Build history of the part. All positions in model axes, mm. Face numbers are marked on the shaded views. A direction names the side the tool comes from. Coordinates: 2 decimals unless noted, no trailing zeros. Loops run counter-clockwise (first coordinate to the right, second up) from the corner with the lowest first, then second, coordinate; pieces in that order, holes last.
(1) Wall check: L1, parallel to Y at x = 35, z = 2.5; L2, parallel to X at y = 50, z = 134; L3, parallel to Y at x = 23, z = 129. Give the ranges that are in metal, low to high.
(2) Slice it at B-B (x = 35). Give the cut face in (y, z).
(3) Two-plate mould, pull along X, no slides. Class the marked faces 4, 5 and 6: pulls with the +X half, pulls with the -X half, needs draft (parallel to the pull), parting line crosses it, or undercut.
(4) Slice it at C-C (z = 112). Give the cut face in (x, y), and give its area (3 significant figures).
(5) Tool access for the marked faces 1, 2 and 3: list every direction of +Z, -Z, +X, -X, +Y, -Y with a clear straight run to the whole face (end or side of a thin tool).
(6) Flat gauge pins, fed straight in: P1, Ø10, axis at x = 7.5, z = 105.5, coming from the +Y side; P2, Ø8, axis at y = 152, z = 72.5, coming from the -X side; P3, Ø24.5, axis at y = 119, z = 119.5, coming from the -X side; P4, Ø6, axis at x = 7, z = 125.5, coming from the +Y side. Where does each tip first touch, or does it go through?
Autodesk Fusion 360 part; units mm, degrees
sketch "Sketch1" plane through (0, 0, 0) normal (0, 1, 0) x (1, 0, 0)
  line L0 (0, 0) -> (70, 0)
  line L1 (70, 0) -> (70, -40)
  line L2 (0, -40) -> (0, 0)
  line L3 (70, -40) -> (12, -40)
  line L4 (70, -90) -> (70, -40)
  line L5 (0, -40) -> (12, -90)
  line L6 (12, -90) -> (12, -140)
  line L7 (12, -140) -> (70, -140)
  line L8 (70, -140) -> (70, -90)
  dimension "d1" = 70
  dimension "d2" = 40
  dimension "d3" = 58
  dimension "d4" = 50
  dimension "d5" = 58
  dimension "d6" = 50
extrude "Extrude1" add sketch "Sketch1" along normal blind 190
sketch "Sketch2" plane through (0, 0, 0) normal (0, 0, -1) x (-1, 0, 0)
  line L0 (-70, 0) -> (0, 0)
  line L1 (0, 0) -> (0, 190)
  line L2 (0, 190) -> (-70, 190)
  line L3 (-70, 190) -> (-70, 0)
sketch "Sketch4" plane through (0, 0, 0) normal (0, 0, -1) x (-1, 0, 0)
  circle A0 centre (-35, 155) radius 25
  line L0 (0, 190) -> (-70, 190)
  line L1 (0, 0) -> (0, 190)
  circle A1 centre (-35, 95) radius 25
  circle A2 centre (-35, 35) radius 25
  dimension "d21" = 50
  dimension "d22" = 35
  dimension "d23" = 35
  dimension "d24" = 50
  dimension "d25" = 35
  dimension "d26" = 60
  dimension "d27" = 50
  dimension "d28" = 35
  dimension "d29" = 60
shell "Shell1" thickness 5 removed faces 1 at (31.3333, 63.3333, 140)
extrude "Extrude2" cut sketch "Sketch4" against normal blind 25
fillet "Fillet1" radius 1 7 edges at (12, 190, 115) (6, 190, 65) (0, 190, 20) (12, 95, 140) (12, 0, 115) (6, 0, 65) (0, 0, 20)
fillet "Fillet2" radius 1 3 edges at (0.2929, 0.2929, 39.9653) (0, 95, 40) (0.2929, 189.7071, 39.9653)
chamfer "Chamfer1" distance 4 angle 45 4 edges at (65, 95, 140) (41, 185, 140) (17, 95, 140) (41, 5, 140)
fillet "Fillet3" radius 0.5 6 edges at (70, 95, 0) (35.5, 190, 0) (0.2929, 189.7071, 0) (0, 95, 0) (0.2929, 0.2929, 0) (35.5, 0, 0)
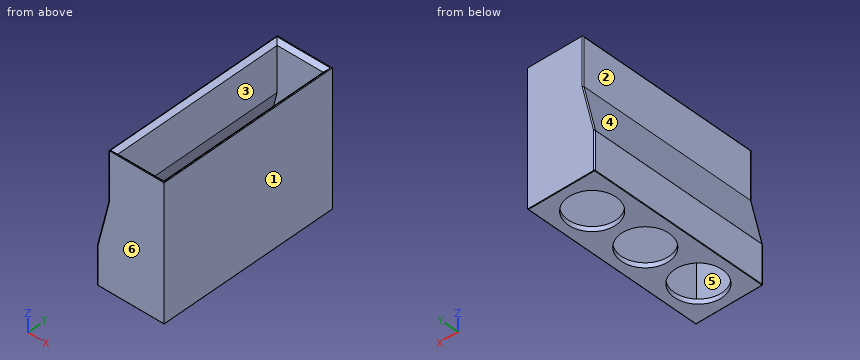
Response values:
1. L1: y = 0 to 10, 60 to 70, 120 to 130, 180 to 190
1. L2: x = 12 to 17, 65 to 70
1. L3: y = 0 to 5, 185 to 190
2. outline: (0, 0.5) arc R0.5 ccw to (0.5, 0) - (10, 0) - (10, 5) - (5, 5) - (5, 136) - (1, 140) - (0, 140) - close; (60, 0) - (70, 0) - (70, 5) - (60, 5) - close; (120, 0) - (130, 0) - (130, 5) - (120, 5) - close; (180, 0) - (189.5, 0) arc R0.5 ccw to (190, 0.5) - (190, 140) - (189, 140) - (185, 136) - (185, 5) - (180, 5) - close
3. face 4: pulls with the -X half
3. face 5: undercut
3. face 6: needs draft
4. outline: (12, 1) arc R1 ccw to (13, 0) - (70, 0) - (70, 190) - (13, 190) arc R1 ccw to (12, 189) - close; hole (17, 5) - (65, 5) - (65, 185) - (17, 185) - close
4. area: 2,380 mm2
5. face 1: +Z, -Z, +X, +Y, -Y
5. face 2: +Z, -X, +Y, -Y
5. face 3: +Z
6. P1: stops at y = 189.87
6. P2: stops at x = 6.84
6. P3: stops at x = 12
6. P4: passes through
